from build123d import *

# Parameters (mm, degrees)
SKETCH1_W               = 35
SKETCH1_H               = 55
SKETCH1_R               = 1.5
SKETCH1_W_2             = 1.053264105
SKETCH1_H_2             = 1.810086697
BOSS_EXTRUDE1_DEPTH     = 3
SKETCH2_W               = 30.130506089
SKETCH2_H               = 18.151203477
BOSS_EXTRUDE2_DEPTH     = 11
SKETCH4_W               = 25.972666726
SKETCH4_H               = 17.735623468
CUT_EXTRUDE2_DEPTH      = 4
CUT_EXTRUDE3_DEPTH      = 36.47534355
CUT_EXTRUDE3_DEPTH_BACK = 36.47534355
SKETCH6_R               = 2.4
CUT_EXTRUDE4_DEPTH      = 35.095454242
CUT_EXTRUDE4_DEPTH_BACK = 2.5
SKETCH7_R               = 3.75


with BuildPart() as part:
    # Sketch1 → Boss-Extrude1 (new body)
    with BuildSketch(Plane(origin=(0, 0, 0), x_dir=(1, 0, 0), z_dir=(0, 1, 0))):
        Rectangle(SKETCH1_W, SKETCH1_H)
        with Locations(Location((14.5, 25, 0), (0, 0, 270))):
            Circle(SKETCH1_R, mode=Mode.SUBTRACT)
        with Locations(Location((-10.5, 25, 0), (0, 0, 270))):
            Circle(SKETCH1_R, mode=Mode.SUBTRACT)
        with Locations(Location((14.5, -25, 0), (0, 0, 270))):
            Circle(SKETCH1_R, mode=Mode.SUBTRACT)
        with Locations(Location((-10.5, -25, 0), (0, 0, 270))):
            Circle(SKETCH1_R, mode=Mode.SUBTRACT)
        with Locations((11.420031076, -18.543755043)):
            Rectangle(SKETCH1_W_2, SKETCH1_H_2, mode=Mode.SUBTRACT)
    extrude(amount=BOSS_EXTRUDE1_DEPTH)

    # Sketch2 → Boss-Extrude2 (add)
    with BuildSketch(Plane(origin=(0, 3, 0), x_dir=(1, 0, 0), z_dir=(0, 1, 0))):
        with Locations((1.371677436, 0.106547158)):
            Rectangle(SKETCH2_W, SKETCH2_H)
    extrude(amount=BOSS_EXTRUDE2_DEPTH)

    # Sketch4 → Cut-Extrude2 (cut)
    with BuildSketch(Plane.XZ):
        with Locations((1.214862274, -0.038232514)):
            Rectangle(SKETCH4_W, SKETCH4_H)
    extrude(amount=-CUT_EXTRUDE2_DEPTH, mode=Mode.SUBTRACT)

    # Sketch6 → Cut-Extrude3 (cut, two sides: drawn at the far end of the back side and taken through both)
    with BuildSketch(Plane.XZ.offset(-CUT_EXTRUDE3_DEPTH_BACK)):
        with Locations(Location((11.63, 3.25, 0), (0, 0, 270))):
            Circle(SKETCH6_R)
        with Locations(Location((-5.17, 5.05, 0), (0, 0, 270))):
            Circle(SKETCH6_R)
        with Locations(Location((-4.17, -3.15, 0), (0, 0, 270))):
            Circle(SKETCH6_R)
        with Locations(Location((6.33, -4.95, 0), (0, 0, 270))):
            Circle(SKETCH6_R)
    extrude(amount=CUT_EXTRUDE3_DEPTH + CUT_EXTRUDE3_DEPTH_BACK, mode=Mode.SUBTRACT)

    # Sketch7 → Cut-Extrude4 (cut, two sides: drawn at the far end of the back side and taken through both)
    with BuildSketch(Plane.XZ.offset(-4).offset(-CUT_EXTRUDE4_DEPTH_BACK)):
        with Locations(Location((-5.17, 5.05, 0), (0, 0, 90))):
            Circle(SKETCH7_R)
        with Locations(Location((-4.17, -3.15, 0), (0, 0, 90))):
            Circle(SKETCH7_R)
        with Locations(Location((6.33, -4.95, 0), (0, 0, 90))):
            Circle(SKETCH7_R)
        with Locations(Location((11.63, 3.25, 0), (0, 0, 46.713081775))):
            Circle(SKETCH7_R)
    extrude(amount=CUT_EXTRUDE4_DEPTH + CUT_EXTRUDE4_DEPTH_BACK, mode=Mode.SUBTRACT)


solid = part.part
Verification items for the finished model (mm, model axes). A direction names the side the tool comes from. Round coordinates to 2 decimals unless told otherwise and drop trailing zeros. Order: outer loops, then holes, each group sorted by start corner. A loop starts at its lowest first (then second) coordinate and runs counter-clockwise, first axis right, second up.
1. Section check D-D on x = -4.17. Record the cut outline in (y, z).
Final values:
outline: (0, -27.5) - (3, -27.5) - (3, -9.18) - (14, -9.18) - (14, -5.55) - (6.5, -5.55) - (6.5, -6.9) - (4, -6.9) - (4, -8.91) - (0, -8.91) - close; (0, 8.83) - (4, 8.83) - (4, 8.66) - (6.5, 8.66) - (6.5, 7.23) - (14, 7.23) - (14, 8.97) - (3, 8.97) - (3, 27.5) - (0, 27.5) - close; (4, 0.6) - (6.5, 0.6) - (6.5, -0.75) - (14, -0.75) - (14, 2.87) - (6.5, 2.87) - (6.5, 1.44) - (4, 1.44) - close
2. Go/stop test with flat-tipped pins: P1, Ø2, axis at x = 11, y = 12.5, coming from the -Z side; P2, Ø4, axis at x = -5.17, z = 5.05, coming from the +Y side; P3, Ø6, axis at x = 11.63, z = 3.25, coming from the +Y side; P4, Ø1.5, axis at x = 1.5, z = -21, coming from the +Y side. Record where each tip stops, or that it passes through.
Final values:
P1: stops at z = -9.18
P2: passes through
P3: stops at y = 14
P4: stops at y = 3
3. Access from +Z, -Z, +X, -X, +Y, -Y to the whole of each face (thin tool, end or side, straight path). Record for faces 3 (the flat face through (10.893, 1, 19)), 4 (the flat face through (1, 8, 8.969)), 5 (the flat face through (-11.771, 2, 0)).
Final values:
face 3: +Y, -Y
face 4: +Z, +X, -X, +Y
face 5: -Y
4. Thickness scan on L1, parallel to X at y = 2.15, z = -25; L2, parallel to Z at x = 6.33, y = 8.5; L3, parallel to Z at x = -2, y = 1. Record the ranges inside material, lowest first.
Final values:
L1: x = -17.5 to -12, -9 to 13, 16 to 17.5
L2: z = -9.18 to -7.35, -2.55 to 8.97
L3: z = -27.5 to -8.91, 8.83 to 27.5
5. Section check A-A on z = 25. Record the cut outline in (x, y).
Final values:
outline: (-17.5, 0) - (-12, 0) - (-12, 3) - (-17.5, 3) - close; (-9, 0) - (13, 0) - (13, 3) - (-9, 3) - close; (16, 0) - (17.5, 0) - (17.5, 3) - (16, 3) - close
6. Release check for a two-part mould opening along X. For faces 1 (the flat face through (1, 14, 0)), 2 (the cylindrical face through (-3.7, 5.3, 8.5)) record: +X half, -X half, draft (parallel to the pull), parting line (faces both ways), or undercut.
Final values:
face 1: draft
face 2: undercut
7. Section check B-B on x = 7. Record the cut outline in (y, z).
Final values:
outline: (0, -27.5) - (3, -27.5) - (3, -9.18) - (14, -9.18) - (14, -7.25) - (6.5, -7.25) - (6.5, -8.64) - (4, -8.64) - (4, -8.91) - (0, -8.91) - close; (0, 8.83) - (4, 8.83) - (4, -1.26) - (6.5, -1.26) - (6.5, -2.65) - (14, -2.65) - (14, 8.97) - (3, 8.97) - (3, 27.5) - (0, 27.5) - close
8. Section check C-C on y = 10. Record the cut outline in (x, z).
Final values:
outline: (-13.69, -9.18) - (16.44, -9.18) - (16.44, 8.97) - (-13.69, 8.97) - close; hole circle Ø4.8 at (-5.17, 5.05); hole circle Ø4.8 at (-4.17, -3.15); hole circle Ø4.8 at (6.33, -4.95); hole circle Ø4.8 at (11.63, 3.25)
